CAD build for the part. Positions are in the model's coordinates, mm. A direction names the side the tool comes from. Round coordinates to 2 decimals unless told otherwise and drop trailing zeros. Order: outer loops, then holes, each group sorted by start corner. A loop starts at its lowest first (then second) coordinate and runs counter-clockwise, first axis right, second up. Notation, with made-up numbers: (15, -33) - (46, -33) arc R32 cw to (46, 5) - close; hole circle Ø2 at (68.5, 83). An arc over 180 degrees is marked (long way). Write item = value, one per line.
from build123d import *

# Parameters (mm, degrees)
SKIZZE1_R                       = 16
AUFSATZ_LINEAR_AUSTRAGEN1_DEPTH = 135
SKIZZE2_R                       = 7.25
AUFSATZ_LINEAR_AUSTRAGEN2_DEPTH = 20
SKIZZE4_R                       = 12.5
AUFSATZ_LINEAR_AUSTRAGEN3_DEPTH = 20
SKIZZE7_R                       = 16
AUFSATZ_LINEAR_AUSTRAGEN4_DEPTH = 10
SKIZZE8_R                       = 17
AUFSATZ_LINEAR_AUSTRAGEN5_DEPTH = 17
SKIZZE9_R                       = 11.376613665
SKIZZE9_R_2                     = 11.354918218
SCHNITT_LINEAR_AUSTRAGEN2_DEPTH = 10
SKIZZE10_R                      = 16
AUFSATZ_LINEAR_AUSTRAGEN6_DEPTH = 20
SKIZZE11_R                      = 5.479403349
SCHNITT_LINEAR_AUSTRAGEN3_DEPTH = 20


with BuildPart() as part:
    # Skizze1 → Aufsatz-Linear austragen1 (new body)
    with BuildSketch(Plane.XY):
        Circle(SKIZZE1_R)
    extrude(amount=AUFSATZ_LINEAR_AUSTRAGEN1_DEPTH)

    # Skizze2 → Aufsatz-Linear austragen2 (add)
    with BuildSketch(Plane(origin=(0, 0, 0), x_dir=(1, 0, 0), z_dir=(0, 1, 0))):
        with Locations(Location((0, -15, 0), (0, 0, 90))):
            Circle(SKIZZE2_R)
    extrude(amount=AUFSATZ_LINEAR_AUSTRAGEN2_DEPTH)

    # Skizze4 → Aufsatz-Linear austragen3 (add)
    with BuildSketch(Plane(origin=(0, 0, 0), x_dir=(1, 0, 0), z_dir=(0, 1, 0))):
        with Locations(Location((0, -41, 0), (0, 0, 90))):
            Circle(SKIZZE4_R)
        with Locations(Location((0, -117, 0), (0, 0, 90))):
            Circle(SKIZZE4_R)
    extrude(amount=AUFSATZ_LINEAR_AUSTRAGEN3_DEPTH)

    # Skizze8 → Aufsatz-Linear austragen5 (add)
    with BuildSketch(Plane(origin=(0, 20, 0), x_dir=(1, 0, 0), z_dir=(0, 1, 0))):
        with Locations(Location((0, -41, 0), (0, 0, 270))):
            Circle(SKIZZE8_R)
        with Locations(Location((0, -117, 0), (0, 0, 270))):
            Circle(SKIZZE8_R)
    extrude(amount=AUFSATZ_LINEAR_AUSTRAGEN5_DEPTH)

    # Skizze9 → Schnitt-Linear austragen2 (cut)
    with BuildSketch(Plane(origin=(0, 37, 0), x_dir=(1, 0, 0), z_dir=(0, 1, 0))):
        with Locations(Location((0, -40.087207053, 0), (0, 0, 270))):
            Circle(SKIZZE9_R)
        with Locations(Location((0, -117.14037352, 0), (0, 0, 270))):
            Circle(SKIZZE9_R_2)
    extrude(amount=-SCHNITT_LINEAR_AUSTRAGEN2_DEPTH, mode=Mode.SUBTRACT)



with BuildPart() as body_2:
    # Skizze7 → Aufsatz-Linear austragen4 (new body)
    with BuildSketch(Plane.XY.offset(135)):
        with BuildLine():
            Line((22.150629915, -17.24109716), (37.5, -7))
            ThreePointArc((37.5, -7), (43.58064746, -0.550964854), (37.446578261, 5.847278882))
            Line((37.446578261, 5.847278882), (22.167008351, 16.063537827))
            ThreePointArc((22.167008351, 16.063537827), (-0.191707942, 27.421836078), (-22.678353656, 16.318958162))
            Line((-22.678353656, 16.318958162), (-37.851181588, 6.422290222))
            ThreePointArc((-37.851181588, 6.422290222), (-44.850742391, -0.656122578), (-37.694365828, -7.575953044))
            Line((-37.694365828, -7.575953044), (-22.830978008, -17.270784777))
            ThreePointArc((-22.830978008, -17.270784777), (-0.332701744, -28.57770368), (22.150629915, -17.24109716))
        make_face()
        Circle(SKIZZE7_R, mode=Mode.SUBTRACT)
    extrude(amount=AUFSATZ_LINEAR_AUSTRAGEN4_DEPTH)


with BuildPart() as part_1:
    add(part.part)

    add(body_2.part)  # Aufsatz-Linear austragen6 merges body 2
    # Skizze10 → Aufsatz-Linear austragen6 (add)
    with BuildSketch(Plane.XY.offset(135)):
        Circle(SKIZZE10_R)
    extrude(amount=AUFSATZ_LINEAR_AUSTRAGEN6_DEPTH)

    # Skizze11 → Schnitt-Linear austragen3 (cut)
    with BuildSketch(Plane.XY.offset(155)):
        Circle(SKIZZE11_R)
    extrude(amount=-SCHNITT_LINEAR_AUSTRAGEN3_DEPTH, mode=Mode.SUBTRACT)


solid = part_1.part
(1) Probe line 1 along Y through (x, z) = (-10, 145.5); line 2 along Z through (x, y) = (23.5, 7.5); line 3 along Y through (x, z) = (-14, 34.5). List the from-to ranges inside material, lowest first.
Solved:
line_1 = -12.49 to 12.49
line_2 = 135 to 145
line_3 = -7.75 to 7.75, 20 to 37
(2) Band-saw the part on C-C on z = 117. List the corners of the cut face in (x, y).
Solved:
outline = (-17, 20) - (-12.5, 20) - (-12.5, 9.99) arc R16 ccw (long way) to (12.5, 9.99) - (12.5, 20) - (17, 20) - (17, 37) - (11.35, 37) - (11.35, 27) - (-11.35, 27) - (-11.35, 37) - (-17, 37) - close
(3) Drop flat-ended pins along their axis: pin 1 (3 mm diameter, centred on x = 11, z = 21.5, fed in from +Y); pin 2 (13.5 mm diameter, centred on x = 0, z = 117.14, fed in from -Y); pin 3 (1.5 mm diameter, centred on x = -14.5, y = 27.5, fed in from +Z). Give the stop position or say it passes through.
Solved:
pin_1 = 12.87
pin_2 = -16
pin_3 = 127
(4) Band-saw the part on D-D on x = 25.5. List the corners of the cut face in (y, z).
Solved:
outline = (-15.01, 135) - (13.84, 135) - (13.84, 145) - (-15.01, 145) - close
(5) Pull direction Z, two halves, no side cores. Call faces 1 (the flat face through (0, 0, 135)), 2 (the cylindrical face through (0.747, 28.381, 100.016)), 3 (the flat face through (0, 0, 0)): released by +Z, released by -Z, zero draft, split by the parting line, or undercut.
Solved:
face_1 = released by +Z
face_2 = undercut
face_3 = released by -Z
(6) Tool access for faces 4 (the cylindrical face through (-3.47, -15.62, 149.93)), 5 (the flat face through (9, 20, 108)), 6 (the cylindrical face through (5.106, 28.381, 57.215)), 7 (the flat face through (7, 0, 155)), 8 (the cylindrical face through (0.172, 27.417, 139.93)): list every direction of +Z, -Z, +X, -X, +Y, -Y with a clear straight run to the whole face (end or side of a thin tool).
Solved:
face_4 = +Z
face_5 = none
face_6 = +Y
face_7 = +Z, +X, -X, +Y, -Y
face_8 = +Z, +Y
(7) Band-saw the part on A-A on z = 46. List the corners of the cut face in (x, y), plus the area to 3 significant figures.
Solved:
outline = (-16.25, 20) - (-11.46, 20) - (-11.46, 11.17) arc R16 ccw (long way) to (11.46, 11.17) - (11.46, 20) - (16.25, 20) - (16.25, 37) - (9.72, 37) - (9.72, 27) - (-9.72, 27) - (-9.72, 37) - (-16.25, 37) - close
area = 1,290 mm²
(8) Band-saw the part on B-B on y = 3.5. List the corners of the cut face in (x, z).
Solved:
outline = (-43.54, 135) - (-15.61, 135) - (-15.61, 0) - (15.61, 0) - (15.61, 135) - (42.12, 135) - (42.12, 145) - (15.61, 145) - (15.61, 155) - (4.22, 155) - (4.22, 135) - (-4.22, 135) - (-4.22, 155) - (-15.61, 155) - (-15.61, 145) - (-43.54, 145) - close
